from build123d import *

# Parameters (mm, degrees)
BASE_FLANGE1_START     = -5
BASE_FLANGE1_OUTLINE_W = 165
BASE_FLANGE1_OUTLINE_H = 120
BASE_FLANGE1_DEPTH     = 5
SKETCH2_R              = 2.75
CUT_EXTRUDE1_DEPTH     = 5
CUT_EXTRUDE2_DEPTH     = 5
FILLET2_R              = 3
SKETCH4_R              = 3
TAB1_DEPTH             = 5
FILLET3_R              = 20


# Read off the part's stored shape, not the designer's step: Base-Flange1
# Sheet-metal steps are written as plain solids
with BuildPart() as part:
    # Base-Flange1 outline → Base-Flange1 (new body)
    with BuildSketch(Plane(origin=(0, 0, 0), x_dir=(1, 0, 0), z_dir=(0, 1, 0)).offset(BASE_FLANGE1_START)):
        Rectangle(BASE_FLANGE1_OUTLINE_W, BASE_FLANGE1_OUTLINE_H)
    extrude(amount=BASE_FLANGE1_DEPTH)

    # Sketch2 → Cut-Extrude1 (cut)
    with BuildSketch(Plane(origin=(0, 0, 0), x_dir=(1, 0, 0), z_dir=(0, 1, 0))):
        with Locations(Location((-72.5, 50, 0), (0, 0, 270))):
            Circle(SKETCH2_R)
        with Locations(Location((-72.5, 0, 0), (0, 0, 270))):
            Circle(SKETCH2_R)
        with Locations(Location((-72.5, -50, 0), (0, 0, 270))):
            Circle(SKETCH2_R)
        with Locations(Location((-27.5, -50, 0), (0, 0, 90))):
            Circle(SKETCH2_R)
        with Locations(Location((-27.5, 0, 0), (0, 0, 90))):
            Circle(SKETCH2_R)
        with Locations(Location((-27.5, 50, 0), (0, 0, 90))):
            Circle(SKETCH2_R)
        with Locations(Location((27.5, -50, 0), (0, 0, 270))):
            Circle(SKETCH2_R)
        with Locations(Location((72.5, -50, 0), (0, 0, 90))):
            Circle(SKETCH2_R)
        with Locations(Location((27.5, 50, 0), (0, 0, 270))):
            Circle(SKETCH2_R)
        with Locations(Location((72.5, 50, 0), (0, 0, 90))):
            Circle(SKETCH2_R)
    extrude(amount=-CUT_EXTRUDE1_DEPTH, mode=Mode.SUBTRACT)

    # Sketch3 → Cut-Extrude2 (cut)
    with BuildSketch(Plane(origin=(0, 0, 0), x_dir=(1, 0, 0), z_dir=(0, 1, 0))):
        Polygon((-62.5, -7.5), (-62.5, -33.99280261), (-24.085436215, -7.5), align=None)
        Polygon((-62.5, 7.5), (-24.085436215, 7.5), (-62.5, 33.99280261), align=None)
        Polygon((-44.789563785, 40), (0, 9.110645666), (44.789563785, 40), align=None)
        Polygon((62.5, 33.99280261), (13.210436215, 0), (62.5, -33.99280261), align=None)
        Polygon((-44.789563785, -40), (44.789563785, -40), (0, -9.110645666), align=None)
    extrude(amount=-CUT_EXTRUDE2_DEPTH, mode=Mode.SUBTRACT)

    # Fillet2
    fillet2_edges = [part.edges().sort_by_distance(p)[0] for p in [
        (13.210436215, -2.5, 0),
        (62.5, -2.5, -33.99280261),
        (62.5, -2.5, 33.99280261),
        (44.789563785, -2.5, 40),
        (-44.789563785, -2.5, 40),
        (0, -2.5, 9.110645666),
        (-62.5, -2.5, 33.99280261),
        (-62.5, -2.5, 7.5),
        (-24.085436215, -2.5, 7.5),
        (-24.085436215, -2.5, -7.5),
        (-62.5, -2.5, -7.5),
        (-62.5, -2.5, -33.99280261),
        (0, -2.5, -9.110645666),
        (-44.789563785, -2.5, -40),
        (44.789563785, -2.5, -40),
    ]]
    fillet(fillet2_edges, radius=FILLET2_R)

    # Sketch4 → Tab1 (add)
    # profile 1 of 4: a face of its own
    with BuildSketch(Plane(origin=(0, 0, 0), x_dir=(1, 0, 0), z_dir=(0, 1, 0))):
        with BuildLine():
            Line((-73.789563785, 60), (-111.742002831, 86.174095894))
            ThreePointArc((-111.742002831, 86.174095894), (-122.174095894, 84.257997169), (-120.257997169, 73.825904106))
            Line((-120.257997169, 73.825904106), (-82.5, 47.785906058))
            Line((-82.5, 47.785906058), (-73.789563785, 60))
        make_face()
        with Locations(Location((-116, 80, 0), (0, 0, 270))):
            Circle(SKETCH4_R, mode=Mode.SUBTRACT)
    # profile 2 of 4: a face of its own
    with BuildSketch(Plane(origin=(0, 0, 0), x_dir=(1, 0, 0), z_dir=(0, 1, 0))):
        with BuildLine():
            Line((73.789563785, 60), (82.5, 47.785906058))
            Line((82.5, 47.785906058), (120.257997169, 73.825904106))
            ThreePointArc((120.257997169, 73.825904106), (122.174095894, 84.257997169), (111.742002831, 86.174095894))
            Line((111.742002831, 86.174095894), (73.789563785, 60))
        make_face()
        with Locations(Location((116, 80, 0), (0, 0, 90))):
            Circle(SKETCH4_R, mode=Mode.SUBTRACT)
    # profile 3 of 4: a face of its own
    with BuildSketch(Plane(origin=(0, 0, 0), x_dir=(1, 0, 0), z_dir=(0, 1, 0))):
        with BuildLine():
            Line((73.789563785, -60), (111.742002831, -86.174095894))
            ThreePointArc((111.742002831, -86.174095894), (122.174095894, -84.257997169), (120.257997169, -73.825904106))
            Line((120.257997169, -73.825904106), (82.5, -47.785906058))
            Line((82.5, -47.785906058), (73.789563785, -60))
        make_face()
        with Locations(Location((116, -80, 0), (0, 0, 270))):
            Circle(SKETCH4_R, mode=Mode.SUBTRACT)
    # profile 4 of 4: a face of its own
    with BuildSketch(Plane(origin=(0, 0, 0), x_dir=(1, 0, 0), z_dir=(0, 1, 0))):
        with BuildLine():
            Line((-73.789563785, -60), (-82.5, -47.785906058))
            Line((-82.5, -47.785906058), (-120.257997169, -73.825904106))
            ThreePointArc((-120.257997169, -73.825904106), (-122.174095894, -84.257997169), (-111.742002831, -86.174095894))
            Line((-111.742002831, -86.174095894), (-73.789563785, -60))
        make_face()
        with Locations(Location((-116, -80, 0), (0, 0, 90))):
            Circle(SKETCH4_R, mode=Mode.SUBTRACT)
    extrude(amount=-TAB1_DEPTH)

    # Fillet3
    fillet3_edges = [part.edges().sort_by_distance(p)[0] for p in [
        (-73.789563785, -2.5, -60),
        (-82.5, -2.5, -47.785906058),
        (82.5, -2.5, -47.785906058),
        (73.789563785, -2.5, -60),
        (73.789563785, -2.5, 60),
        (82.5, -2.5, 47.785906058),
        (-82.5, -2.5, 47.785906058),
        (-73.789563785, -2.5, 60),
    ]]
    fillet(fillet3_edges, radius=FILLET3_R)


solid = part.part
Can you work these out from the model? Positions are in its coordinate system, mm. A direction names the side the tool comes from. Give positions to 0.01 mm unless a question says otherwise; leave off trailing zeros. Loops run counter-clockwise (first coordinate to the right, second up) from the corner with the lowest first, then second, coordinate; pieces in that order, holes last. Notation, with made-up numbers: (79.5, -12.75) -> (114.5, -12.75) arc R18 ccw to (114.5, -5.75) -> close; hole circle Ø9 at (40, 42.5). An arc over 180 degrees is marked (long way). Return JSON: item names as keys, results as strings.
Q1. On a 3-axis mill with a long thin cutter (end or side, diameter ignored), from which of +Z, -Z, +X, -X, +Y, -Y can I reach the whole of each face in a straight line? I mean faces 1 (the face through (0, -2, 40)), 2 (the face through (82.5, -3, 1)). Say none if no direction works.
Checks:
{"face 1": "+Y, -Y", "face 2": "+X, +Y, -Y"}
Q2. For pin 1 Ø2 at (x, y) = (30, -1.5) entering from -Z; pin 2 Ø1.5 at (y, z) = (-3, -4) entering from +X; pin 3 Ø1.5 at (y, z) = (-3, 4.5) entering from -X, each with a flat end and sliding along its axis, tell me the tip position at first contact or that it passes through.
Checks:
{"pin 1": "stops at z = -60", "pin 2": "stops at x = 82.5", "pin 3": "stops at x = -82.5"}
Q3. I want a section at D-D, the plane x = 72.5. List the corners of the cut face in (y, z) for me.
Checks:
{"outline": "(-5, -60.62) -> (0, -60.62) -> (0, -52.75) -> (-5, -52.75) -> close; (-5, -47.25) -> (0, -47.25) -> (0, 47.25) -> (-5, 47.25) -> close; (-5, 52.75) -> (0, 52.75) -> (0, 60.62) -> (-5, 60.62) -> close"}
Q4. I need wall thicknesses on probe 1 along X at (y, z) = (-3.9, 0); probe 2 along X at (y, z) = (-1.15, 80); probe 3 along X at (y, z) = (-3, 50). Which ranges of each line are inside material? Lowest first, please.
Checks:
{"probe 1": "x = -82.5 to -75.25, -69.75 to -30.25, -24.75 to 15.49, 62.5 to 82.5", "probe 2": "x = -123.5 to -119, -113 to -102.79, 102.79 to 113, 119 to 123.5", "probe 3": "x = -87.06 to -75.25, -69.75 to -30.25, -24.75 to 24.75, 30.25 to 69.75, 75.25 to 87.06"}
Q5. We'd pull the mould along X, two halves only. Please class faces 3 (the face through (113.97, -2.46, -77.79)), 4 (the face through (84.73, -2.54, 46.46)), 5 (the face through (-105.91, -2.46, -63.93)), 6 (the face through (-70.641, -2.465, -52.027)): released by +X, released by -X, zero draft, split by the parting line, or undercut.
Checks:
{"face 3": "undercut", "face 4": "released by +X", "face 5": "released by -X", "face 6": "undercut"}
Q6. I want a section at C-C, the plane x = 116. List the corners of the cut face in (y, z) for me, then the cut area to 3 significant figures.
Checks:
{"outline": "(-5, -87.5) -> (0, -87.5) -> (0, -83) -> (-5, -83) -> close; (-5, -77) -> (0, -77) -> (0, -70.89) -> (-5, -70.89) -> close; (-5, 70.89) -> (0, 70.89) -> (0, 77) -> (-5, 77) -> close; (-5, 83) -> (0, 83) -> (0, 87.5) -> (-5, 87.5) -> close", "area": "106 mm2"}
Q7. I want a section at B-B, the plane z = -80. List the corners of the cut face in (x, y) for me, then the cut area to 3 significant figures.
Checks:
{"outline": "(-123.5, -5) -> (-119, -5) -> (-119, 0) -> (-123.5, 0) -> close; (-113, -5) -> (-102.79, -5) -> (-102.79, 0) -> (-113, 0) -> close; (102.79, -5) -> (113, -5) -> (113, 0) -> (102.79, 0) -> close; (119, -5) -> (123.5, -5) -> (123.5, 0) -> (119, 0) -> close", "area": "147 mm2"}
Q8. I want a section at A-A, the plane x = 27.5. List the corners of the cut face in (y, z) for me.
Checks:
{"outline": "(-5, -60) -> (0, -60) -> (0, -52.75) -> (-5, -52.75) -> close; (-5, -47.25) -> (0, -47.25) -> (0, -40) -> (-5, -40) -> close; (-5, -28.08) -> (0, -28.08) -> (0, -9.85) -> (-5, -9.85) -> close; (-5, 9.85) -> (0, 9.85) -> (0, 28.08) -> (-5, 28.08) -> close; (-5, 40) -> (0, 40) -> (0, 47.25) -> (-5, 47.25) -> close; (-5, 52.75) -> (0, 52.75) -> (0, 60) -> (-5, 60) -> close"}
